```python
from build123d import *

# Parameters (mm, degrees)
SKETCH048_W           = 9.7
SKETCH048_H           = 50
SKETCH048_R           = 4
SKETCH048_R_2         = 2.5
PAD028_DEPTH          = 5
SKETCH049_W           = 1
SKETCH049_H           = 5.04
POCKET023_DEPTH       = 5.001
SKETCH050_R           = 1.5
POCKET024_DEPTH       = 9.701
CLONE_PLACEMENT_ANGLE = 90


with BuildPart() as part:
    # Sketch048 → Pad028 (new body)
    with BuildSketch(Plane.XY):
        Rectangle(SKETCH048_W, SKETCH048_H)
        with Locations((0, -16.25)):
            Circle(SKETCH048_R, mode=Mode.SUBTRACT)
        with Locations((0, 15)):
            Circle(SKETCH048_R_2, mode=Mode.SUBTRACT)
    extrude(amount=PAD028_DEPTH)

    # Sketch049 (on Face8 of Pad028) → Pocket023 (cut, through all)
    with BuildSketch(Plane.XY.offset(5)):
        with Locations((0, -22.48)):
            Rectangle(SKETCH049_W, SKETCH049_H)
    extrude(amount=-POCKET023_DEPTH, mode=Mode.SUBTRACT)

    # Sketch050 (on Face3 of Pocket023) → Pocket024 (cut, through all)
    with BuildSketch(Plane.YZ.offset(4.85)):
        with Locations((-22.5, 2.5)):
            Circle(SKETCH050_R)
    extrude(amount=-POCKET024_DEPTH, mode=Mode.SUBTRACT)


with BuildPart() as part_1:
    # Clone placement: moved
    add(part.part.moved(Location((-326, 1, 493))).rotate(Axis((-326, 1, 493), (0, 0, 1)), CLONE_PLACEMENT_ANGLE))


with BuildPart() as part_2:
    # Clone044 placement: moved
    add(part_1.part.moved(Location((0, -410, 0))))


solid = part_2.part
```
CAD build for the part. Positions are in the model's coordinates, mm. A direction names the side the tool comes from. Give positions to 0.01 mm unless a question says otherwise; leave off trailing zeros. Write each loop counter-clockwise with the first axis right and the second up, starting at its lowest first coordinate (ties: lowest second). Pieces come first, ordered by that corner, then holes. Notation, with made-up numbers: (-35.5, 42) -> (-28.5, 42) arc R23 cw to (-28.5, 50) -> close; hole circle Ø3 at (82, 74). An arc over 180 degrees is marked (long way). Write each question's results on one line, items separated by ' | '.
1. Cut at D-D, the plane x = -309.75. Write the cut outline in (y, z), then the cut area to 3 significant figures.
Geometry check:
outline: (-413.85, 493) -> (-413, 493) -> (-413, 498) -> (-413.85, 498) -> close; (-405, 493) -> (-404.15, 493) -> (-404.15, 498) -> (-405, 498) -> close | area: 8.50 mm²
2. Two-plate mould, pull along Y, no slides. Class faces 3 (the flat face through (-302, -409.5, 494)), 4 (the flat face through (-326, -413.85, 495)), 5 (the flat face through (-326, -404.15, 495)), 6 (the flat face through (-326, -409, 493)): pulls with the +Y half, pulls with the -Y half, needs draft (parallel to the pull), parting line crosses it, or undercut.
Geometry check:
face 3: undercut | face 4: pulls with the -Y half | face 5: pulls with the +Y half | face 6: needs draft
3. Cut at B-B, the plane z = 495.5. Write the cut outline in (x, y).
Geometry check:
outline: (-351, -413.85) -> (-305, -413.85) -> (-305, -409.5) -> (-305.78, -409.5) arc R4 cw (long way) to (-305.78, -408.5) -> (-305, -408.5) -> (-305, -404.15) -> (-351, -404.15) -> close; (-302, -413.85) -> (-301, -413.85) -> (-301, -409.5) -> (-302, -409.5) -> close; (-302, -408.5) -> (-301, -408.5) -> (-301, -404.15) -> (-302, -404.15) -> close; hole circle Ø5 at (-341, -409)
4. Cut at A-A, the plane y = -409. Write the cut outline in (x, z).
Geometry check:
outline: (-351, 493) -> (-343.5, 493) -> (-343.5, 498) -> (-351, 498) -> close; (-338.5, 493) -> (-313.75, 493) -> (-313.75, 498) -> (-338.5, 498) -> close
5. Which spindle directions (+Z, -Z, +X, -X, +Y, -Y) get a long thin tool onto all of the face, cutting with end or side? Do faces 1 (the flat face through (-302, -408.5, 494)), 2 (the cylindrical face through (-313.746, -408.831, 495.465)). Say none if no direction does.
Geometry check:
face 1: +Z, -Z, +X | face 2: +Z, -Z
6. Cut at C-C, the plane x = -303.5. Write the cut outline in (y, z).
Geometry check:
outline: (-413.85, 493) -> (-409.5, 493) -> (-409.5, 494) -> (-413.85, 494) -> close; (-413.85, 497) -> (-409.5, 497) -> (-409.5, 498) -> (-413.85, 498) -> close; (-408.5, 493) -> (-404.15, 493) -> (-404.15, 494) -> (-408.5, 494) -> close; (-408.5, 497) -> (-404.15, 497) -> (-404.15, 498) -> (-408.5, 498) -> close
7. Wall check: probe 1 along X at (y, z) = (-411, 495.25); probe 2 along X at (y, z) = (-407.1, 495.5); probe 3 along X at (y, z) = (-409, 495.4). Give the ranges that are in metal, low to high. Write a range as [from, to].
Geometry check:
probe 1: [-351, -342.5], [-339.5, -313.21], [-306.29, -304.98], [-302.02, -301] | probe 2: [-351, -342.62], [-339.38, -313.27], [-306.23, -305], [-302, -301] | probe 3: [-351, -343.5], [-338.5, -313.75]
